from build123d import *

# Parameters (mm, degrees)
SKETCH_1_R           = 51.5
SKETCH_1_R_2         = 25
EXTRUDE_1_DEPTH      = 9
CUT_EXTRUDE_START    = -8
SKETCH_12_R          = 51.5
SKETCH_12_R_2        = 50
CUT_EXTRUDE_11_DEPTH = 8
SKETCH_3_W           = 54
SKETCH_3_H           = 75
CUT_EXTRUDE_2_DEPTH  = 74.385965961
CHAMFER_1_SIZE       = 4
SKETCH_4_R           = 46.5
CUT_EXTRUDE_3_DEPTH  = 3
SKETCH_7_R           = 1.5
CUT_EXTRUDE_6_DEPTH  = 74.385965961
SKETCH_8_R           = 3
CUT_EXTRUDE_7_DEPTH  = 3
SKETCH_11_W          = 65
SKETCH_11_H          = 72
CUT_EXTRUDE_10_DEPTH = 74.385965961
FILLET_1_R           = 5.5
SKETCH_13_R          = 1.5
CUT_EXTRUDE_12_DEPTH = 20
SKETCH_14_R          = 3
CUT_EXTRUDE_13_DEPTH = 3


with BuildPart() as part:
    # 草图1 → 凸台-拉伸1 (new body)
    with BuildSketch(Plane(origin=(0, 0, 0), x_dir=(1, 0, 0), z_dir=(0, 1, 0))):
        with Locations(Location((0, 0, 0), (0, 0, 270))):
            Circle(SKETCH_1_R)
        with Locations(Location((0, 0, 0), (0, 0, 270))):
            Circle(SKETCH_1_R_2, mode=Mode.SUBTRACT)
    extrude(amount=EXTRUDE_1_DEPTH)

    # 草图12 → 切除-拉伸11 (cut)
    with BuildSketch(Plane(origin=(0, 9, 0), x_dir=(1, 0, 0), z_dir=(0, 1, 0)).offset(CUT_EXTRUDE_START)):
        with Locations(Location((0, 0, 0), (0, 0, 270))):
            Circle(SKETCH_12_R)
        with Locations(Location((0, 0, 0), (0, 0, 270))):
            Circle(SKETCH_12_R_2, mode=Mode.SUBTRACT)
    extrude(amount=CUT_EXTRUDE_11_DEPTH, mode=Mode.SUBTRACT)

    # 草图3 → 切除-拉伸2 (cut, through all)
    with BuildSketch(Plane(origin=(0, 9, 0), x_dir=(1, 0, 0), z_dir=(0, 1, 0))):
        Rectangle(SKETCH_3_W, SKETCH_3_H)
    extrude(amount=-CUT_EXTRUDE_2_DEPTH, mode=Mode.SUBTRACT)

    # 倒角1
    chamfer_1_edges = [part.edges().sort_by_distance(p)[0] for p in [
        (0, 9, -37.5),
        (0, 9, 37.5),
    ]]
    chamfer(chamfer_1_edges, length=CHAMFER_1_SIZE)

    # 草图4 → 切除-拉伸3 (cut)
    with BuildSketch(Plane.XZ):
        with Locations(Location((0, 0, 0), (0, 0, 270))):
            Circle(SKETCH_4_R)
    extrude(amount=-CUT_EXTRUDE_3_DEPTH, mode=Mode.SUBTRACT)

    # 草图7 → 切除-拉伸6 (cut, through all)
    with BuildSketch(Plane.XZ):
        with Locations(Location((0, 46.5, 0), (0, 0, 270))):
            Circle(SKETCH_7_R)
        with Locations(Location((40.270181276, 23.25, 0), (0, 0, 270))):
            Circle(SKETCH_7_R)
        with Locations(Location((40.270181276, -23.25, 0), (0, 0, 270))):
            Circle(SKETCH_7_R)
        with Locations(Location((0, -46.5, 0), (0, 0, 270))):
            Circle(SKETCH_7_R)
        with Locations(Location((-40.270181276, -23.25, 0), (0, 0, 270))):
            Circle(SKETCH_7_R)
        with Locations(Location((-40.270181276, 23.25, 0), (0, 0, 270))):
            Circle(SKETCH_7_R)
    extrude(amount=-CUT_EXTRUDE_6_DEPTH, mode=Mode.SUBTRACT)

    # 草图8 → 切除-拉伸7 (cut)
    with BuildSketch(Plane.XZ):
        with Locations((0, 46.5)):
            Circle(SKETCH_8_R)
        with Locations((40.270181276, 23.25)):
            Circle(SKETCH_8_R)
        with Locations((40.270181276, -23.25)):
            Circle(SKETCH_8_R)
        with Locations((0, -46.5)):
            Circle(SKETCH_8_R)
        with Locations((-40.270181276, -23.25)):
            Circle(SKETCH_8_R)
        with Locations((-40.270181276, 23.25)):
            Circle(SKETCH_8_R)
    extrude(amount=-CUT_EXTRUDE_7_DEPTH, mode=Mode.SUBTRACT)

    # 草图11 → 切除-拉伸10 (cut, through all)
    with BuildSketch(Plane(origin=(0, 9, 0), x_dir=(1, 0, 0), z_dir=(0, 1, 0))):
        Rectangle(SKETCH_11_W, SKETCH_11_H)
    extrude(amount=-CUT_EXTRUDE_10_DEPTH, mode=Mode.SUBTRACT)

    # 圆角1
    # the kernel refuses this fillet: 5.5 mm, written as the material it adds along each edge
    with BuildSketch(Plane(origin=(-32.5, 9, 36), x_dir=(1, 0, 0), z_dir=(0, -1, 0))) as fillet_1_piece_1_section:
        with BuildLine():
            CenterArc((FILLET_1_R, -FILLET_1_R), FILLET_1_R, 90, 90)
            Line((0, -FILLET_1_R), (0, 0))
            Line((0, 0), (FILLET_1_R, 0))
        make_face()
    fillet_1_piece_1 = extrude(amount=9, mode=Mode.PRIVATE)
    fillet_1_piece_1 = split(fillet_1_piece_1, bisect_by=Plane(origin=(-30.907548225, 3, 34.407548225), z_dir=(0, 1, 0)), keep=Keep.TOP, mode=Mode.PRIVATE)
    fillet_1_piece_1 = fillet_1_piece_1 & Plane(origin=(0, 6, 0), x_dir=(0, 0, -1), z_dir=(0, -1, 0)) * Cylinder(46.5, 40, mode=Mode.PRIVATE)
    add(fillet_1_piece_1)
    with BuildSketch(Plane(origin=(-32.5, 9, 36), x_dir=(1, 0, 0), z_dir=(0, -1, 0))) as fillet_1_piece_2_section:
        with BuildLine():
            CenterArc((FILLET_1_R, -FILLET_1_R), FILLET_1_R, 90, 90)
            Line((0, -FILLET_1_R), (0, 0))
            Line((0, 0), (FILLET_1_R, 0))
        make_face()
    fillet_1_piece_2 = extrude(amount=9, mode=Mode.PRIVATE)
    fillet_1_piece_2 = split(fillet_1_piece_2, bisect_by=Plane(origin=(-31.523516263, 3, 35.138738602), z_dir=(0, 1, 0)), keep=Keep.TOP, mode=Mode.PRIVATE)
    fillet_1_piece_2 = fillet_1_piece_2 - Plane(origin=(0, 6, 0), x_dir=(0, 0, -1), z_dir=(0, -1, 0)) * Cylinder(46.5, 40, mode=Mode.PRIVATE)
    add(fillet_1_piece_2)
    with BuildSketch(Plane(origin=(-32.5, 9, 36), x_dir=(1, 0, 0), z_dir=(0, -1, 0))) as fillet_1_piece_3_section:
        with BuildLine():
            CenterArc((FILLET_1_R, -FILLET_1_R), FILLET_1_R, 90, 90)
            Line((0, -FILLET_1_R), (0, 0))
            Line((0, 0), (FILLET_1_R, 0))
        make_face()
    fillet_1_piece_3 = extrude(amount=9, mode=Mode.PRIVATE)
    fillet_1_piece_3 = split(fillet_1_piece_3, bisect_by=Plane(origin=(-31.523516263, 3, 35.138738602), z_dir=(0, -1, 0)), keep=Keep.TOP, mode=Mode.PRIVATE)
    fillet_1_piece_3 = fillet_1_piece_3 - Plane(origin=(0, 1.5, 0), x_dir=(0, 0, -1), z_dir=(0, -1, 0)) * Cylinder(46.5, 40, mode=Mode.PRIVATE)
    add(fillet_1_piece_3)
    with BuildSketch(Plane(origin=(32.5, 9, 36), x_dir=(-1, 0, 0), z_dir=(0, -1, 0))) as fillet_1_piece_4_section:
        with BuildLine():
            CenterArc((FILLET_1_R, FILLET_1_R), FILLET_1_R, 180, 90)
            Line((0, FILLET_1_R), (0, 0))
            Line((0, 0), (FILLET_1_R, 0))
        make_face()
    fillet_1_piece_4 = extrude(amount=9, mode=Mode.PRIVATE)
    fillet_1_piece_4 = split(fillet_1_piece_4, bisect_by=Plane(origin=(30.907548225, 3, 34.407548225), z_dir=(0, 1, 0)), keep=Keep.TOP, mode=Mode.PRIVATE)
    fillet_1_piece_4 = fillet_1_piece_4 & Plane(origin=(0, 6, 0), x_dir=(0, 0, -1), z_dir=(0, -1, 0)) * Cylinder(46.5, 40, mode=Mode.PRIVATE)
    add(fillet_1_piece_4)
    with BuildSketch(Plane(origin=(32.5, 9, 36), x_dir=(-1, 0, 0), z_dir=(0, -1, 0))) as fillet_1_piece_5_section:
        with BuildLine():
            CenterArc((FILLET_1_R, FILLET_1_R), FILLET_1_R, 180, 90)
            Line((0, FILLET_1_R), (0, 0))
            Line((0, 0), (FILLET_1_R, 0))
        make_face()
    fillet_1_piece_5 = extrude(amount=9, mode=Mode.PRIVATE)
    fillet_1_piece_5 = split(fillet_1_piece_5, bisect_by=Plane(origin=(31.523516263, 3, 35.138738602), z_dir=(0, 1, 0)), keep=Keep.TOP, mode=Mode.PRIVATE)
    fillet_1_piece_5 = fillet_1_piece_5 - Plane(origin=(0, 6, 0), x_dir=(0, 0, -1), z_dir=(0, -1, 0)) * Cylinder(46.5, 40, mode=Mode.PRIVATE)
    add(fillet_1_piece_5)
    with BuildSketch(Plane(origin=(32.5, 9, 36), x_dir=(-1, 0, 0), z_dir=(0, -1, 0))) as fillet_1_piece_6_section:
        with BuildLine():
            CenterArc((FILLET_1_R, FILLET_1_R), FILLET_1_R, 180, 90)
            Line((0, FILLET_1_R), (0, 0))
            Line((0, 0), (FILLET_1_R, 0))
        make_face()
    fillet_1_piece_6 = extrude(amount=9, mode=Mode.PRIVATE)
    fillet_1_piece_6 = split(fillet_1_piece_6, bisect_by=Plane(origin=(31.523516263, 3, 35.138738602), z_dir=(0, -1, 0)), keep=Keep.TOP, mode=Mode.PRIVATE)
    fillet_1_piece_6 = fillet_1_piece_6 - Plane(origin=(0, 1.5, 0), x_dir=(0, 0, -1), z_dir=(0, -1, 0)) * Cylinder(46.5, 40, mode=Mode.PRIVATE)
    add(fillet_1_piece_6)
    with BuildSketch(Plane(origin=(32.5, 9, -36), x_dir=(0, 0, 1), z_dir=(0, -1, 0))) as fillet_1_piece_7_section:
        with BuildLine():
            CenterArc((FILLET_1_R, FILLET_1_R), FILLET_1_R, 180, 90)
            Line((0, FILLET_1_R), (0, 0))
            Line((0, 0), (FILLET_1_R, 0))
        make_face()
    fillet_1_piece_7 = extrude(amount=9, mode=Mode.PRIVATE)
    fillet_1_piece_7 = fillet_1_piece_7 & Plane(origin=(0, 6, 0), x_dir=(0, 0, -1), z_dir=(0, -1, 0)) * Cylinder(46.5, 40, mode=Mode.PRIVATE)
    fillet_1_piece_7 = split(fillet_1_piece_7, bisect_by=Plane(origin=(30.907548225, 3, -34.407548225), z_dir=(0, 1, 0)), keep=Keep.TOP, mode=Mode.PRIVATE)
    add(fillet_1_piece_7)
    with BuildSketch(Plane(origin=(32.5, 9, -36), x_dir=(0, 0, 1), z_dir=(0, -1, 0))) as fillet_1_piece_8_section:
        with BuildLine():
            CenterArc((FILLET_1_R, FILLET_1_R), FILLET_1_R, 180, 90)
            Line((0, FILLET_1_R), (0, 0))
            Line((0, 0), (FILLET_1_R, 0))
        make_face()
    fillet_1_piece_8 = extrude(amount=9, mode=Mode.PRIVATE)
    fillet_1_piece_8 = fillet_1_piece_8 - Plane(origin=(0, 6, 0), x_dir=(0, 0, -1), z_dir=(0, -1, 0)) * Cylinder(46.5, 40, mode=Mode.PRIVATE)
    fillet_1_piece_8 = split(fillet_1_piece_8, bisect_by=Plane(origin=(31.523516263, 3, -35.138738602), z_dir=(0, 1, 0)), keep=Keep.TOP, mode=Mode.PRIVATE)
    add(fillet_1_piece_8)
    with BuildSketch(Plane(origin=(32.5, 9, -36), x_dir=(0, 0, 1), z_dir=(0, -1, 0))) as fillet_1_piece_9_section:
        with BuildLine():
            CenterArc((FILLET_1_R, FILLET_1_R), FILLET_1_R, 180, 90)
            Line((0, FILLET_1_R), (0, 0))
            Line((0, 0), (FILLET_1_R, 0))
        make_face()
    fillet_1_piece_9 = extrude(amount=9, mode=Mode.PRIVATE)
    fillet_1_piece_9 = fillet_1_piece_9 - Plane(origin=(0, 1.5, 0), x_dir=(0, 0, -1), z_dir=(0, -1, 0)) * Cylinder(46.5, 40, mode=Mode.PRIVATE)
    fillet_1_piece_9 = split(fillet_1_piece_9, bisect_by=Plane(origin=(31.523516263, 3, -35.138738602), z_dir=(0, -1, 0)), keep=Keep.TOP, mode=Mode.PRIVATE)
    add(fillet_1_piece_9)
    with BuildSketch(Plane(origin=(-32.5, 9, -36), x_dir=(1, 0, 0), z_dir=(0, -1, 0))) as fillet_1_piece_10_section:
        with BuildLine():
            CenterArc((FILLET_1_R, FILLET_1_R), FILLET_1_R, 180, 90)
            Line((0, FILLET_1_R), (0, 0))
            Line((0, 0), (FILLET_1_R, 0))
        make_face()
    fillet_1_piece_10 = extrude(amount=9, mode=Mode.PRIVATE)
    fillet_1_piece_10 = fillet_1_piece_10 & Plane(origin=(0, 6, 0), x_dir=(0, 0, -1), z_dir=(0, -1, 0)) * Cylinder(46.5, 40, mode=Mode.PRIVATE)
    fillet_1_piece_10 = split(fillet_1_piece_10, bisect_by=Plane(origin=(-30.907548225, 3, -34.407548225), z_dir=(0, 1, 0)), keep=Keep.TOP, mode=Mode.PRIVATE)
    add(fillet_1_piece_10)
    with BuildSketch(Plane(origin=(-32.5, 9, -36), x_dir=(1, 0, 0), z_dir=(0, -1, 0))) as fillet_1_piece_11_section:
        with BuildLine():
            CenterArc((FILLET_1_R, FILLET_1_R), FILLET_1_R, 180, 90)
            Line((0, FILLET_1_R), (0, 0))
            Line((0, 0), (FILLET_1_R, 0))
        make_face()
    fillet_1_piece_11 = extrude(amount=9, mode=Mode.PRIVATE)
    fillet_1_piece_11 = fillet_1_piece_11 - Plane(origin=(0, 6, 0), x_dir=(0, 0, -1), z_dir=(0, -1, 0)) * Cylinder(46.5, 40, mode=Mode.PRIVATE)
    fillet_1_piece_11 = split(fillet_1_piece_11, bisect_by=Plane(origin=(-31.523516263, 3, -35.138738602), z_dir=(0, 1, 0)), keep=Keep.TOP, mode=Mode.PRIVATE)
    add(fillet_1_piece_11)
    with BuildSketch(Plane(origin=(-32.5, 9, -36), x_dir=(1, 0, 0), z_dir=(0, -1, 0))) as fillet_1_piece_12_section:
        with BuildLine():
            CenterArc((FILLET_1_R, FILLET_1_R), FILLET_1_R, 180, 90)
            Line((0, FILLET_1_R), (0, 0))
            Line((0, 0), (FILLET_1_R, 0))
        make_face()
    fillet_1_piece_12 = extrude(amount=9, mode=Mode.PRIVATE)
    fillet_1_piece_12 = fillet_1_piece_12 - Plane(origin=(0, 1.5, 0), x_dir=(0, 0, -1), z_dir=(0, -1, 0)) * Cylinder(46.5, 40, mode=Mode.PRIVATE)
    fillet_1_piece_12 = split(fillet_1_piece_12, bisect_by=Plane(origin=(-31.523516263, 3, -35.138738602), z_dir=(0, -1, 0)), keep=Keep.TOP, mode=Mode.PRIVATE)
    add(fillet_1_piece_12)

    # 草图13 → 切除-拉伸12 (cut)
    with BuildSketch(Plane(origin=(90.573916545, 17, 197.95666402), x_dir=(0.9918515590673906, 0, 0.1273989198368124), z_dir=(0, 1, 0))):
        with Locations(Location((-161.529552035, 187.909140098, 0), (0, 0, 277.319311568))):
            Circle(SKETCH_13_R)
        with Locations(Location((-153.594739562, 188.928331456, 0), (0, 0, 277.319311568))):
            Circle(SKETCH_13_R)
        with Locations(Location((-159.236371478, 170.055812034, 0), (0, 0, 277.319311568))):
            Circle(SKETCH_13_R)
        with Locations(Location((-151.301559005, 171.075003393, 0), (0, 0, 277.319311568))):
            Circle(SKETCH_13_R)
        with Locations(Location((-79.850576146, 198.400441146, 0), (0, 0, 277.319311568))):
            Circle(SKETCH_13_R)
        with Locations(Location((-71.915763673, 199.419632505, 0), (0, 0, 277.319311568))):
            Circle(SKETCH_13_R)
        with Locations(Location((-77.557395589, 180.547113083, 0), (0, 0, 277.319311568))):
            Circle(SKETCH_13_R)
        with Locations(Location((-69.622583116, 181.566304442, 0), (0, 0, 277.319311568))):
            Circle(SKETCH_13_R)
    extrude(amount=-CUT_EXTRUDE_12_DEPTH, mode=Mode.SUBTRACT)

    # 草图14 → 切除-拉伸13 (cut)
    with BuildSketch(Plane.XZ):
        with Locations((-45.7, 9)):
            Circle(SKETCH_14_R)
        with Locations((44.65, 9)):
            Circle(SKETCH_14_R)
        with Locations((-45.7, -9)):
            Circle(SKETCH_14_R)
        with Locations((44.65, -9)):
            Circle(SKETCH_14_R)
    extrude(amount=-CUT_EXTRUDE_13_DEPTH, mode=Mode.SUBTRACT)


solid = part.part
Check sheet for the modelled part. Datum: model origin and axes. Units: mm. A direction names the side the tool comes from. Coordinates: 2 decimals unless noted, no trailing zeros. Loops run counter-clockwise (first coordinate to the right, second up) from the corner with the lowest first, then second, coordinate; pieces in that order, holes last. Notation, with made-up numbers: (82, 20.5) -> (99, 20.5) arc R11 cw to (99, 38.5) -> close; hole circle Ø9 at (-5.75, 41). An arc over 180 degrees is marked (long way). Write item = value, one per line. Start each with the question number.
1. Depth check by flat-ended pin: P1, Ø3.5, axis at x = 44.65, z = -9, coming from the -Y side; P2, Ø5, axis at y = 6.5, z = 30, coming from the -X side; P3, Ø2.5, axis at x = 36.65, z = 9, coming from the -Y side; P4, Ø3.5, axis at x = 36.65, z = -9, coming from the +Y side. Enter the tip coordinate at first touch or a pass-through.
2. Section check C-C on z = 23.25. Record the cut outline in (x, y), then the cut area to 3 significant figures.
3. Section check B-B on z = 0. Record the cut outline in (x, y), then the cut area to 3 significant figures.
4. Section check D-D on x = 36.65. Record the cut outline in (y, z).
5. Material ranges on line 1 (Z direction, x = -37.7, y = 7.4); line 2 (X direction, y = 4.85, z = -23.25); line 3 (X direction, y = 5.5, z = 0), recorded low to high.
6. Draft check along X on faces 4 (the cylindrical face through (15.02, 4.94, 47.69)), 5 (the cylindrical face through (-0.1, 1.5, -49.5)), 6 (the flat face through (8, 0, 46)). Enter one of: released by +X, released by -X, zero draft, split by the parting line, or undercut.
7. Tool access check on faces 1 (the cylindrical face through (-30.93, 6.04, -34.35)), 2 (the cylindrical face through (-48.63, 1.48, 9.65)), 3 (the flat face through (-27, 7, 38)). Record the directions out of +Z, -Z, +X, -X, +Y, -Y that give a thin tool (end or side, any length) a straight path to the whole face; none if there is none.
8. Section check A-A on x = 0. Record the cut outline in (y, z), then the cut area to 3 significant figures.
Responses:
q1.P1 = 3
q1.P2 = -41.76
q1.P3 = through
q1.P4 = 9
q2.outline = (-45.95, 0) -> (-43.27, 0) -> (-43.27, 3) -> (-41.77, 3) -> (-41.77, 9) -> (-44.27, 9) -> (-44.27, 1) -> (-45.95, 1) -> close; (-38.77, 3) -> (-32.5, 3) -> (-32.5, 9) -> (-38.77, 9) -> close; (32.5, 3) -> (38.77, 3) -> (38.77, 9) -> (32.5, 9) -> close; (41.77, 3) -> (43.27, 3) -> (43.27, 0) -> (45.95, 0) -> (45.95, 1) -> (44.27, 1) -> (44.27, 9) -> (41.77, 9) -> close
q2.area = 115 mm2
q3.outline = (-51.5, 0) -> (-46.5, 0) -> (-46.5, 3) -> (-32.5, 3) -> (-32.5, 9) -> (-50, 9) -> (-50, 1) -> (-51.5, 1) -> close; (32.5, 3) -> (46.5, 3) -> (46.5, 0) -> (51.5, 0) -> (51.5, 1) -> (50, 1) -> (50, 9) -> (32.5, 9) -> close
q3.area = 234 mm2
q4.outline = (0, -36.18) -> (1, -36.18) -> (1, -34.01) -> (9, -34.01) -> (9, -10.5) -> (3, -10.5) -> (3, -28.62) -> (0, -28.62) -> close; (0, 28.62) -> (3, 28.62) -> (3, 10.5) -> (9, 10.5) -> (9, 34.01) -> (1, 34.01) -> (1, 36.18) -> (0, 36.18) -> close; (3, -7.5) -> (9, -7.5) -> (9, 7.5) -> (3, 7.5) -> close
q5.line_1 = -32.84 to -10.5, -7.5 to 7.5, 10.5 to 32.84
q5.line_2 = -44.27 to -41.77, -38.77 to -32.5, 32.5 to 38.77, 41.77 to 44.27
q5.line_3 = -50 to -32.5, 32.5 to 50
q6.face_4 = split by the parting line
q6.face_5 = undercut
q6.face_6 = zero draft
q7.face_1 = +Y, -Y
q7.face_2 = -Y
q7.face_3 = +Y
q8.outline = (0, -51.5) -> (1, -51.5) -> (1, -50) -> (9, -50) -> (9, -48) -> (3, -48) -> (3, -49.5) -> (0, -49.5) -> close; (0, 49.5) -> (3, 49.5) -> (3, 48) -> (9, 48) -> (9, 50) -> (1, 50) -> (1, 51.5) -> (0, 51.5) -> close; (3, -45) -> (9, -45) -> (9, -41.5) -> (5, -37.5) -> (3, -37.5) -> close; (3, 37.5) -> (5, 37.5) -> (9, 41.5) -> (9, 45) -> (3, 45) -> close
q8.area = 104 mm2
